Check sheet for the modelled part. Datum: model origin and axes. Units: mm. Face numbers are marked on the shaded views. Give positions to 0.01 mm unless a question says otherwise; leave off trailing zeros. Order: outer loops, then holes, each group sorted by start corner. A loop starts at its lowest first (then second) coordinate and runs counter-clockwise, first axis right, second up.
Item 1: Sectioned sample at D-D on x = 6. Record the boundary of the cut face in (y, z) (3 decimals), and give its area (3 significant figures).
Item 2: Sectioned sample at C-C on y = -3. Record the boundary of the cut face in (x, z).
Item 3: Sectioned sample at A-A on z = 8. Count the separate pieces of the cut face and the enclosed holes in it, and give its area (3 significant figures).
Item 4: Release check for a two-part mould opening along X. For the marked faces 1, 2, 3 and 4 record: released by +X, released by -X, zero draft, split by the parting line, or undercut.
Item 5: Sectioned sample at B-B on x = -8.75. Record the boundary of the cut face in (y, z) (3 decimals), and give its area (3 significant figures).
Item 6: Material ranges on line 1 along X through (y, z) = (4, 10.25); line 2 along X through (y, z) = (4.25, 8.5); line 3 along Z through (x, y) = (-7.25, 0.5), recorded low to high.
Item 7: Gauge pin test, flat ends, axial feed: P1, Ø4, axis at y = 4.5, z = 6.5, coming from the -X side; P2, Ø3, axis at y = -1.5, z = 8.5, coming from the +X side; P3, Ø0.8, axis at x = 10.5, y = 6.5, coming from the +Z side; P4, Ø5, axis at x = 6, z = 12, coming from the +Y side (3 decimals). Record the tip position at first contact, or that the pin passes through.
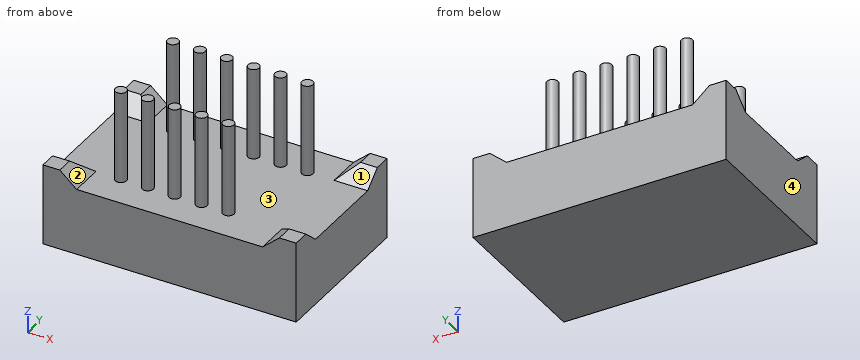
from build123d import *

# Parameters (mm, degrees)
F0_W     = 22.6
F0_H     = 14.07
F1_DEPTH = 7.24
F3_DEPTH = 25
F5_DEPTH = 25
F6_R     = 0.5
F7_DEPTH = 8.18


with BuildPart() as f1:
    # F0 (on Top) → F1 (new body)
    with BuildSketch(Plane.XY):
        Rectangle(F0_W, F0_H)
    extrude(amount=F1_DEPTH)

    # F2 (on face) → F3 (cut)
    with BuildSketch(Plane.XZ.offset(7.035)):
        Polygon((0, 7.24), (-9.8, 7.24), (-8.3, 5.94), (0, 5.94), (8.3, 5.94), (9.8, 7.24), align=None)
    extrude(amount=-F3_DEPTH, mode=Mode.SUBTRACT)

    # F4 (on face) → F5 (cut)
    with BuildSketch(Plane(origin=(-11.3, 0, 0), x_dir=(0, -1, 0), z_dir=(-1, 0, 0))):
        Polygon((0, 7.24), (-5.535, 7.24), (-4.035, 5.94), (0, 5.94), (4.035, 5.94), (5.535, 7.24), align=None)
    extrude(amount=-F5_DEPTH, mode=Mode.SUBTRACT)

    # F6 (on face) → F7 (join)
    with BuildSketch(Plane.XY.offset(5.94)):
        with Locations((-6.073824, -4.035)):
            Circle(F6_R)
        with Locations((-6.073824, 4.035)):
            Circle(F6_R)
        with Locations((-3.673824, 4.035)):
            Circle(F6_R)
        with Locations((-1.273824, 4.035)):
            Circle(F6_R)
        with Locations((1.126176, 4.035)):
            Circle(F6_R)
        with Locations((3.526176, 4.035)):
            Circle(F6_R)
        with Locations((5.926176, 4.035)):
            Circle(F6_R)
        with Locations((-3.673824, -4.035)):
            Circle(F6_R)
        with Locations((-1.273824, -4.035)):
            Circle(F6_R)
        with Locations((1.126176, -4.035)):
            Circle(F6_R)
        with Locations((3.526176, -4.035)):
            Circle(F6_R)
    extrude(amount=F7_DEPTH)


solid = f1.part
Report:
1. outline: (-7.035, 0) - (7.035, 0) - (7.035, 5.94) - (4.53, 5.94) - (4.53, 14.12) - (3.54, 14.12) - (3.54, 5.94) - (-7.035, 5.94) - close
1. area: 91.7 mm2
2. outline: (-11.3, 0) - (11.3, 0) - (11.3, 5.94) - (-11.3, 5.94) - close
3. separate pieces: 11
3. enclosed holes: 0
3. area: 8.64 mm2
4. face 1: zero draft
4. face 2: undercut
4. face 3: undercut
4. face 4: released by -X
5. outline: (-7.035, 0) - (7.035, 0) - (7.035, 6.33) - (4.485, 6.33) - (4.035, 5.94) - (-4.035, 5.94) - (-4.485, 6.33) - (-7.035, 6.33) - close
5. area: 85.7 mm2
6. line 1: x = -6.57 to -5.58, -4.17 to -3.18, -1.77 to -0.78, 0.63 to 1.62, 3.03 to 4.02, 5.43 to 6.42
6. line 2: x = -6.53 to -5.62, -4.13 to -3.22, -1.73 to -0.82, 0.67 to 1.58, 3.07 to 3.98, 5.47 to 6.38
6. line 3: z = 0 to 5.94
7. P1: stops at x = -11.3
7. P2: passes through
7. P3: stops at z = 7.24
7. P4: stops at y = 4.535
